The listing builds one solid part. Answer for the finished solid, in the listing's coordinates (mm). A direction names the side the tool comes from. Give positions to 0.01 mm unless a question says otherwise; leave off trailing zeros. Write each loop counter-clockwise with the first axis right and the second up, starting at its lowest first coordinate (ties: lowest second). Pieces come first, ordered by that corner, then holes. Notation, with made-up numbers: (26, -30.5) - (32, -30.5) arc R25 cw to (32, 7.5) - close; hole circle Ø3 at (-39.75, 28). An arc over 180 degrees is marked (long way). Answer in a Markdown table with one row per item. Add a question column.
from build123d import *

# Parameters (mm, degrees)
BOSS_EXTRUDE1_DEPTH = 3


with BuildPart() as part:
    # Sketch2 → Boss-Extrude1 (new body)
    with BuildSketch(Plane(origin=(0, 0, 0), x_dir=(1, 0, 0), z_dir=(0, 1, 0))):
        with BuildLine():
            Line((-15.860247962, 17.20906431), (-13.694996915, 20.301363277))
            ThreePointArc((-13.694996915, 20.301363277), (-19.875283017, 22.25), (-26.055569119, 20.301363277))
            Line((-26.055569119, 20.301363277), (-26.055569119, 33.889213566))
            Line((-26.055569119, 33.889213566), (26.055569119, 33.889213566))
            Line((26.055569119, 33.889213566), (26.055569119, 20.301363277))
            ThreePointArc((26.055569119, 20.301363277), (19.875283017, 22.25), (13.694996915, 20.301363277))
            Line((13.694996915, 20.301363277), (15.860247962, 17.20906431))
            ThreePointArc((15.860247962, 17.20906431), (13.666207185, 14.707240293), (12.875283017, 11.475))
            ThreePointArc((12.875283017, 11.475), (10.090653959, 8.727908609), (6.180286102, 8.826363277))
            ThreePointArc((6.180286102, 8.826363277), (0, 10.775), (-6.180286102, 8.826363277))
            ThreePointArc((-6.180286102, 8.826363277), (-10.090653959, 8.727908609), (-12.875283017, 11.475))
            ThreePointArc((-12.875283017, 11.475), (-13.666207185, 14.707240293), (-15.860247962, 17.20906431))
        make_face()
    extrude(amount=BOSS_EXTRUDE1_DEPTH)


solid = part.part
1. A tool of negligible diameter and unlimited length cuts with its end or side. For faces 5 (the face through (-19.78, 1.48, -22.25)), 6 (the face through (-14.793, 1.479, -18.734)), 7 (the face through (0.092, 1.479, -10.775)), from which of +Z, -Z, +X, -X, +Y, -Y can it reach the whole face along a straight path? Write none if from no direction.
2. Section D-D (z = -12) is taken. Give the vertices of the cut face in (x, y) (3 decimals).
3. Section B-B (y = 1.3) is taken. Give the vertices of the cut face in (x, z) (3 decimals), and give its area (3 significant figures).
4. Section A-A (z = -21.25) is taken. Give the vertices of the cut face in (x, y).
5. The mould has two halves that part along Z. Classify faces 1 (the face through (10.143, 1.479, -8.749)), 2 (the face through (-26.056, 1, -27)), 3 (the face through (0, 1, -33.889)), 4 (the face through (14.76, 1.48, -18.78)): +Z half, -Z half, draft (parallel to the pull), parting line (faces both ways), or undercut.
6. Section C-C (x = -4.5) is taken. Give the vertices of the cut face in (y, z).
7. Straight lines are drawn through the part: L1, parallel to X at y = 0.75, z = -14.75; L2, parallel to Z at x = -15, y = 1.2; L3, parallel to Z at x = -21, y = 0.75. For each, find the intervals that lie inside material, in ascending order. Write a range as [from, to].
Geometry check:
| question | item | result |
|---|---|---|
| 1 | face 5 | +Y, -Y |
| 1 | face 6 | -X, +Y, -Y |
| 1 | face 7 | +Z, +Y, -Y |
| 2 | outline | (-12.895, 0) - (12.895, 0) - (12.895, 3) - (-12.895, 3) - close |
| 3 | outline | (-26.056, -33.889) - (26.056, -33.889) - (26.056, -20.301) arc R10.775 cw to (13.695, -20.301) - (15.86, -17.209) arc R7 cw to (12.875, -11.475) arc R5 ccw to (6.18, -8.826) arc R10.775 cw to (-6.18, -8.826) arc R5 ccw to (-12.875, -11.475) arc R7 cw to (-15.86, -17.209) - (-13.695, -20.301) arc R10.775 cw to (-26.056, -20.301) - close |
| 3 | area | 974 mm² |
| 4 | outline | (-26.06, 0) - (-24.41, 0) - (-24.41, 3) - (-26.06, 3) - close; (-15.34, 0) - (15.34, 0) - (15.34, 3) - (-15.34, 3) - close; (24.41, 0) - (26.06, 0) - (26.06, 3) - (24.41, 3) - close |
| 5 | face 1 | +Z half |
| 5 | face 2 | draft |
| 5 | face 3 | -Z half |
| 5 | face 4 | undercut |
| 6 | outline | (0, -33.89) - (3, -33.89) - (3, -9.79) - (0, -9.79) - close |
| 7 | L1 | [-13.69, 13.69] |
| 7 | L2 | [-33.89, -21.08], [-18.44, -16.5] |
| 7 | L3 | [-33.89, -22.19] |
